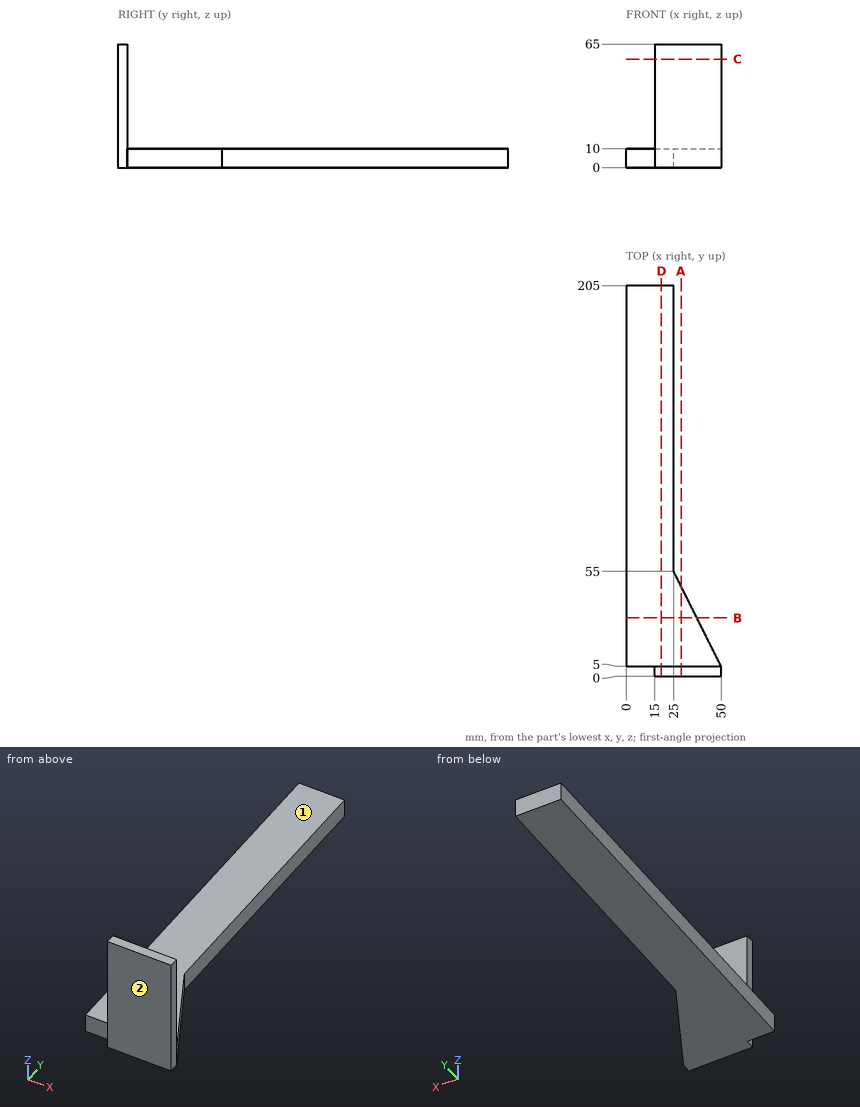
Can you work these out from the drawing? Everything is in mm from the part's minimum corner. A direction names the side the tool comes from. Coordinates: 2 decimals unless noted, no trailing zeros. Write each loop counter-clockwise with the first axis right and the second up, starting at its lowest first coordinate (ties: lowest second). Pieces come first, ordered by that corner, then holes. Notation, with made-up numbers: (83, 34) -> (132, 34) arc R25 cw to (132, 71) -> close; hole circle Ø4 at (3, -2.5). An arc over 180 degrees is marked (long way). Write item = value, one per line.
(1) Imagine slicing it at D-D (x = 18.5). Please give me the cut outline in (y, z), and give its area (4 significant figures).
Verdict:
outline = (0, 0) -> (205, 0) -> (205, 10) -> (5, 10) -> (5, 65) -> (0, 65) -> close
area = 2,325 mm^2
(2) Imagine slicing it at A-A (x = 29). Please give me the cut outline in (y, z).
Verdict:
outline = (0, 0) -> (47, 0) -> (47, 10) -> (5, 10) -> (5, 65) -> (0, 65) -> close
(3) If I drill on probe 1 along Z at (x, y) = (7, 131); probe 2 along Y at (x, z) = (20, 19.5); probe 3 along X at (y, z) = (150.5, 6.5), over which ranges is the centre line in solid material (lowest first)?
Verdict:
probe_1 = 0 to 10
probe_2 = 0 to 5
probe_3 = 0 to 25
(4) Imagine slicing it at B-B (y = 30.5). Please give me the cut outline in (x, z), and give its area (4 significant figures).
Verdict:
outline = (0, 0) -> (37.25, 0) -> (37.25, 10) -> (0, 10) -> close
area = 372.5 mm^2
(5) Imagine slicing it at C-C (z = 57). Please give me the cut outline in (x, y), and give its area (3 significant figures).
Verdict:
outline = (15, 0) -> (50, 0) -> (50, 5) -> (15, 5) -> close
area = 175 mm^2
(6) On a 3-axis mill with a long thin cutter (end or side, diameter ignored), from which of +Z, -Z, +X, -X, +Y, -Y can I reach the whole of each face in a straight line? I mean the marked faces 1 and 2. Say none if no direction works.
Verdict:
face_1 = +Z, +X, -X, +Y
face_2 = +Z, -Z, +X, -X, -Y
(7) For pin 1 (5 mm diameter, centred on y = 142.5, z = 4, fed in from +X); pin 2 (25 mm diameter, centred on x = 31.5, y = 57.5, fed in from +Z); pin 3 (3 mm diameter, centred on x = 28, y = 152.5, fed in from -Z); pin 4 (2.5 mm diameter, centred on y = 2.5, z = 35, fed in from -X), each with a flat end and sliding along its axis, tell me the tip position at first contact or that it passes through.
Verdict:
pin_1 = 25
pin_2 = 10
pin_3 = through
pin_4 = 15
